Could you check a few things on this drawing? It's one solid part, dimensions in mm from its lowest x, y, z. Give positions to 0.01 mm unless a question says otherwise; leave off trailing zeros. Loops run counter-clockwise (first coordinate to the right, second up) from the corner with the lowest first, then second, coordinate; pieces in that order, holes last.
1. I need wall thicknesses on line 1 along Z through (x, y) = (5, 0.7); line 2 along Y through (x, z) = (15, 17.6); line 3 along X through (y, z) = (3.5, 2.1). Which ranges of each line are inside material? Lowest first, please.
2. For P1, Ø1.8, axis at x = 5, z = 16, coming from the +Y side (1 decimal); P2, Ø1.2, axis at y = 0.5, z = 11, coming from the +X side, each with a flat end and sliding along its axis, tell me the tip position at first contact or that it passes through.
3. Imagine slicing it at C-C (z = 4). List the corners of the cut face in (x, y) for me (1 decimal), plus the area to 3 significant figures.
4. Imagine slicing it at B-B (x = 5). List the corners of the cut face in (y, z) for me (1 decimal).
5. Thinking about a two-plate mould opening in Z: for the marked faces 1, 2 and 3, which applies, +Z half, -Z half, draft (parallel to the pull), parting line (faces both ways), or undercut?
6. Imagine slicing it at A-A (y = 3.5). List the corners of the cut face in (x, z) for me, plus the area to 3 significant figures.
7. Imagine slicing it at D-D (x = 13.75). List the corners of the cut face in (y, z) for me.
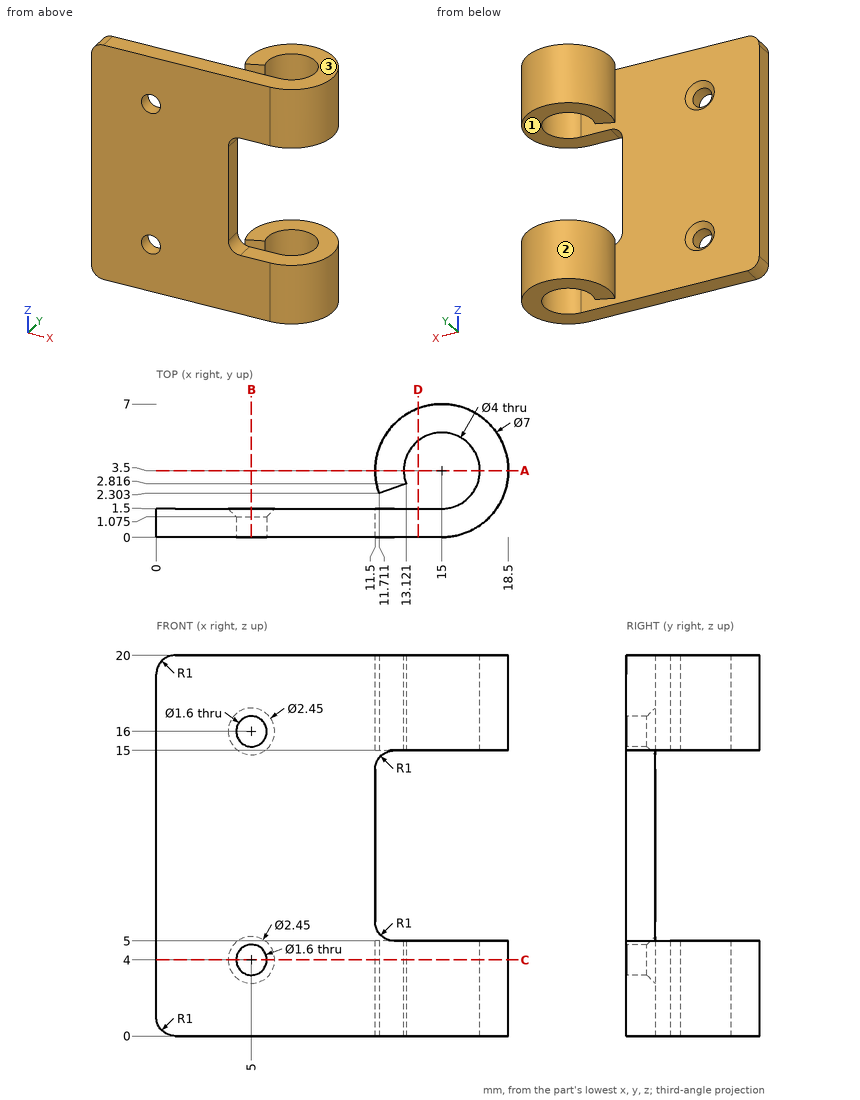
Derived:
1. line 1: z = 0 to 3.2, 4.8 to 15.2, 16.8 to 20
1. line 2: y = 0 to 1.5, 5.5 to 7
1. line 3: x = 11.5 to 13, 17 to 18.5
2. P1: stops at y = 1.2
2. P2: stops at x = 11.5
3. outline: (0, 0) - (4.2, 0) - (4.2, 1.1) - (3.8, 1.5) - (0, 1.5) - close; (5.8, 0) - (15, 0) arc R3.5 ccw (long way) to (11.7, 2.3) - (13.1, 2.8) arc R2 cw (long way) to (15, 1.5) - (6.2, 1.5) - (5.8, 1.1) - close
3. area: 40.8 mm2
4. outline: (0, 0) - (1.5, 0) - (1.5, 2.8) - (1.1, 3.2) - (0, 3.2) - close; (0, 4.8) - (1.1, 4.8) - (1.5, 5.2) - (1.5, 14.8) - (1.1, 15.2) - (0, 15.2) - close; (0, 16.8) - (1.1, 16.8) - (1.5, 17.2) - (1.5, 20) - (0, 20) - close
5. face 1: undercut
5. face 2: draft
5. face 3: +Z half
6. outline: (11.5, 0) - (13, 0) - (13, 5) - (11.5, 5) - close; (11.5, 15) - (13, 15) - (13, 20) - (11.5, 20) - close; (17, 0) - (18.5, 0) - (18.5, 5) - (17, 5) - close; (17, 15) - (18.5, 15) - (18.5, 20) - (17, 20) - close
6. area: 30.0 mm2
7. outline: (0, 0) - (1.5, 0) - (1.5, 5) - (0, 5) - close; (0, 15) - (1.5, 15) - (1.5, 20) - (0, 20) - close; (5.06, 0) - (6.77, 0) - (6.77, 5) - (5.06, 5) - close; (5.06, 15) - (6.77, 15) - (6.77, 20) - (5.06, 20) - close
